The listing builds one solid part. Answer for the finished solid, in the listing's coordinates (mm). Face numbers are marked on the shaded views. A direction names the side the tool comes from. Give positions to 0.01 mm unless a question says otherwise; leave off trailing zeros. Order: outer loops, then holes, each group sorted by start corner. A loop starts at its lowest first (then second) coordinate and runs counter-clockwise, first axis right, second up. Notation, with made-up numbers: (-5, 12) - (3, 12) arc R17 ccw to (3, 24) - close; hole circle Ø4 at (14, 32). An arc over 180 degrees is marked (long way). Answer as CSV lines item,"result". Start each with the question number.
1. Consider line 1 along X through (y, z) = (-7, 52); line 2 along X through (y, z) = (4, 67.5); line 3 along Y through (x, z) = (11.1, 13.4). Determine where each line is inside the solid, lowest interval first. Write a range as [from, to].
2. Determine the mould class of the marked faces 1, 2 and 3 for opening direction X: +X half, -X half, draft (parallel to the pull), parting line (faces both ways), or undercut.
3. Section D-D on y = 7 is taken. Give the vertices of the cut face in (x, z).
4. Section A-A on z = 13.4 is taken. Give the vertices of the cut face in (x, y), and give its area (3 significant figures).
5. Section C-C on x = -6 is taken. Give the vertices of the cut face in (y, z), and give its area (3 significant figures).
6. Which of the six approach directions +Z, -Z, +X, -X, +Y, -Y give full straight-line access (tool end or side, diameter ignored) to the marked faces 4 and 5?
7. Section B-B on z = 39 is taken. Give the vertices of the cut face in (x, y).
8. Flat-ended cylindrical pins translate along their axes: pin 1 (10 mm diameter, centred on y = -3, z = 91, fed in from -X); pin 2 (7 mm diameter, centred on y = -1, z = 15.5, fed in from +X); pin 3 (1.1 mm diameter, centred on x = 13, z = 14, fed in from -Y); pin 4 (0.7 mm diameter, centred on x = 12.5, z = 13.5, fed in from +Y). Find the tip coordinate at first contact, or state that the pin passes through.
Autodesk Inventor part; units mm, degrees
ref_plane "Work Plane2" through (0, 9.7015, 84.25) normal (0.7660444, 0, 0.6427876) x (0, -1, 0)
ref_plane "YZ Plane" through (0, 0, 0) normal (1, 0, 0) x (0, 1, 0)
ref_plane "XZ Plane" through (0, 0, 0) normal (0, 1, 0) x (-1, 0, 0)
sketch "Sketch1" plane through (0, 0, 0) normal (0, 0, 1) x (1, 0, 0)
  line L0 (-12.4, 10.5) -> (12.4, 10.5)
  line L1 (12.4, 10.5) -> (12.4, -10.5)
  line L2 (12.4, -10.5) -> (-12.4, -10.5)
  line L3 (-12.4, -10.5) -> (-12.4, 10.5)
  point P0 (0, 0)
  point P1 (-12.4, 0)
  point P2 (0, 10.5)
  dimension "d0" = 24.8
  dimension "d1" = 21
extrude "Extrusion1" add sketch "Sketch1" along normal blind 1.75
ref_plane "Work Plane1" through (0, 0, 84.25) normal (0, 0, 1) x (1, 0, 0)
sketch "Sketch3" plane through (0, 0, 84.25) normal (0, 0, 1) x (1, 0, 0)
  line L0 (0, 9.7015) -> (0, -9.7015) construction
  point P0 (0, 0)
  point P1 (0, 0)
ref_plane "Work Plane2" through (0, 9.7015, 84.25) normal (0.7660444, 0, 0.6427876) x (0, -1, 0)
sketch "Sketch2" plane through (0, 0, 1.75) normal (0, 0, 1) x (1, 0, 0)
  line L0 (12.4, 10.5) -> (12.4, -10.5)
  line L1 (-12.4, 10.5) -> (12.4, 10.5)
  line L2 (12.4, -10.5) -> (-12.4, -10.5)
  line L3 (-12.4, 10.5) -> (-10.65, 10.5)
  line L4 (-10.65, 10.5) -> (-10.65, -10.5)
  line L5 (-10.65, -10.5) -> (-12.4, -10.5)
  line L6 (-12.4, -10.5) -> (-12.4, 10.5)
  line L7 (12.4, -10.5) -> (10.65, -10.5)
  line L8 (10.65, -10.5) -> (10.65, 10.5)
  line L9 (10.65, 10.5) -> (12.4, 10.5)
  line L10 (12.4, 10.5) -> (12.4, -10.5)
  point P0 (0, 0)
  dimension "d4" = 1.75
  dimension "d5" = 1.75
extrude "Extrusion2" add sketch "Sketch2" along normal up to surface contours L0 L2 L8 L1 | L4 L2 L6 L1 surface through (0, 9.7015, 84.25) normal (0.7660444, 0, 0.6427876)
sketch "Sketch4" plane through (-12.4, -10.5, 0) normal (0, -1, 0) x (1, 0, 0)
  line L0 (1.75, 96.9422) -> (0, 99.0277)
  line L1 (24.8, 69.4723) -> (23.05, 71.5578)
  line L2 (23.05, 1.75) -> (23.05, 71.5578)
  line L3 (23.05, 71.5578) -> (23.05, 74.2803)
  line L4 (23.05, 74.2803) -> (39.014, 55.2552)
  line L5 (39.014, 55.2552) -> (37.6734, 54.1303)
  line L6 (37.6734, 54.1303) -> (24.8, 69.4723)
  line L7 (0, 99.0277) -> (-12.8734, 114.3697)
  line L8 (-12.8734, 114.3697) -> (-11.5328, 115.4946)
  line L9 (-11.5328, 115.4946) -> (1.75, 99.6647)
  line L10 (1.75, 99.6647) -> (1.75, 96.9422)
  line L11 (24.8, 0) -> (24.8, 69.4723)
  line L12 (23.05, 71.5578) -> (23.05, 74.2803)
  line L13 (23.05, 74.2803) -> (1.75, 99.6647)
  line L14 (1.75, 99.6647) -> (1.75, 96.9422)
  line L15 (1.75, 96.9422) -> (23.05, 71.5578)
  point P0 (12.4, 0)
  dimension "d10" = 1.75
  dimension "d11" = 22.75
  dimension "d12" = 1.75
  dimension "d13" = 22.75
extrude "Extrusion3" add sketch "Sketch4" against normal up to surface (21 mm away)
sketch "Sketch5" plane through (-10.65, -10.5, 1.75) normal (1, 0, 0) x (0, 0, -1)
  line L0 (0, 0) -> (-95.1922, 0)
  line L1 (0, 21) -> (-23.3, 21)
  line L2 (-23.3, 21) -> (-23.3, 0)
  line L3 (-23.3, 0) -> (0, 0)
  line L4 (0, 0) -> (0, 21)
  circle A0 centre (-11.65, 10.5) radius 1.7
  point P0 (-97.7359, 0)
  point P1 (1.75, 10.5)
  dimension "d16" = 23.3
  dimension "d17" = 3.4
extrude "Extrusion4" cut sketch "Sketch5" against normal up to surface (1.75 mm away) contours A0
mirror "Mirror1" about plane through (0, 0, 0) normal (1, 0, 0) of "Extrusion4"
sketch "Sketch8" plane through (-23.9328, -10.5, 115.4946) normal (0.7660444, 0, 0.6427876) x (0.6427876, 0, -0.7660444)
  line L0 (0, 0) -> (0, 21)
  line L1 (78.6369, 0) -> (78.6369, 21)
  circle A0 centre (10.5, 10.5) radius 1.7
  circle A1 centre (68.1369, 10.5) radius 1.7
  point P0 (103.8577, 10.5)
  point P1 (0, 10.5)
  point P2 (78.6369, 10.5)
  dimension "d25" = 3.4
  dimension "d26" = 3.4
  dimension "d27" = 10.5
  dimension "d28" = 10.5
extrude "Extrusion6" cut sketch "Sketch8" against normal up to surface (1.75 mm away)
sketch "Sketch9" plane through (-12.4, -10.5, 99.0277) normal (-0.7660444, 0, -0.6427876) x (-0.6427876, 0, 0.7660444)
  circle A0 centre (9.5275, 10.5) radius 1.7
  line L0 (20.0275, 21) -> (0, 21)
  circle A1 centre (9.5275, 10.5) radius 4.3
  line L1 (11.1441, 7.7) -> (7.9109, 7.7)
  line L2 (7.9109, 7.7) -> (6.2943, 10.5)
  line L3 (6.2943, 10.5) -> (7.9109, 13.3)
  line L4 (7.9109, 13.3) -> (11.1441, 13.3)
  line L5 (11.1441, 13.3) -> (12.7606, 10.5)
  line L6 (12.7606, 10.5) -> (11.1441, 7.7)
  circle A2 centre (-48.1094, 10.5) radius 1.7
  line L7 (-38.582, 21) -> (-58.6094, 21)
  circle A3 centre (-48.1094, 10.5) radius 4.3
  line L8 (-46.4929, 7.7) -> (-49.726, 7.7)
  line L9 (-49.726, 7.7) -> (-51.3426, 10.5)
  line L10 (-51.3426, 10.5) -> (-49.726, 13.3)
  line L11 (-49.726, 13.3) -> (-46.4929, 13.3)
  line L12 (-46.4929, 13.3) -> (-44.8763, 10.5)
  line L13 (-44.8763, 10.5) -> (-46.4929, 7.7)
  point P0 (-83.8302, 10.5)
  dimension "d31" = 5.6
  dimension "d32" = 1.5
  dimension "d38" = 5.6
  dimension "d39" = 1.5
extrude "Extrusion7" cut sketch "Sketch9" against normal blind 0.75 contours L1 L2 L3 L4 L5 L6
extrude "Extrusion8" add sketch "Sketch9" along normal blind 1.55 contours A1
draft "FaceDraft1" angle 45 pull direction (-0.7660444, 0, -0.6427876) faces at (-22.0708, -0.346, 108.9453) fixed edges at (-16.9475, 0, 102.0359)
extrude "Extrusion9" cut sketch "Sketch9" against normal blind 0.75 contours L8 L9 L10 L11 L12 L13
extrude "Extrusion10" add sketch "Sketch9" along normal blind 1.55 contours A3
draft "FaceDraft2" angle 45 pull direction (-0.7660444, 0, -0.6427876) faces at (15.0044, -0.6898, 64.7609) fixed edges at (20.1008, 0, 57.8835)
sketch "Sketch10" plane through (12.4, -10.5, 0) normal (1, 0, 0) x (0, 0, -1)
  circle A0 centre (-13.4, 10.5) radius 1.7
  line L0 (0, 21) -> (-69.4723, 21)
  circle A1 centre (-13.4, 10.5) radius 4.3
  line L1 (-11.7834, 7.7) -> (-15.0166, 7.7)
  line L2 (-15.0166, 7.7) -> (-16.6332, 10.5)
  line L3 (-16.6332, 10.5) -> (-15.0166, 13.3)
  line L4 (-15.0166, 13.3) -> (-11.7834, 13.3)
  line L5 (-11.7834, 13.3) -> (-10.1668, 10.5)
  line L6 (-10.1668, 10.5) -> (-11.7834, 7.7)
  point P0 (0, 10.5)
  dimension "d45" = 5.6
  dimension "d46" = 1.5
extrude "Extrusion11" cut sketch "Sketch10" against normal blind 0.75 contours L1 L2 L3 L4 L5 L6
extrude "Extrusion12" add sketch "Sketch10" along normal blind 1.55 contours A1
draft "FaceDraft3" angle 45 pull direction (1, 0, 0) faces at (12.9167, -0.6898, 9.1557) fixed edges at (13.95, 0, 17.7)
sketch "Sketch11" plane through (-10.65, -10.5, 1.75) normal (1, 0, 0) x (0, 0, -1)
  line L0 (0, 0) -> (-95.1922, 0)
  line L1 (0, 21) -> (0, 0)
  line L2 (0, 21) -> (-95.1922, 21)
  line L3 (-25.35, 21) -> (-23.6, 21)
  line L4 (-23.6, 21) -> (-23.6, 0)
  line L5 (-23.6, 0) -> (-25.35, 0)
  line L6 (-25.35, 0) -> (-25.35, 21)
  point P0 (1.75, 10.5)
  dimension "d52" = 1.75
  dimension "d53" = 23.6
extrude "Extrusion13" add sketch "Sketch11" along normal blind 3 contours L0 L6 L2 L4
mirror "Mirror2" about plane through (0, 0, 0) normal (1, 0, 0) of "Extrusion13"
equation "\"d4\" = d5"
equation "\"d12\" = d10"
equation "\"d26\" = d25"
equation "\"d28\" = d27"
properties part number "carousel_mount_bracket"
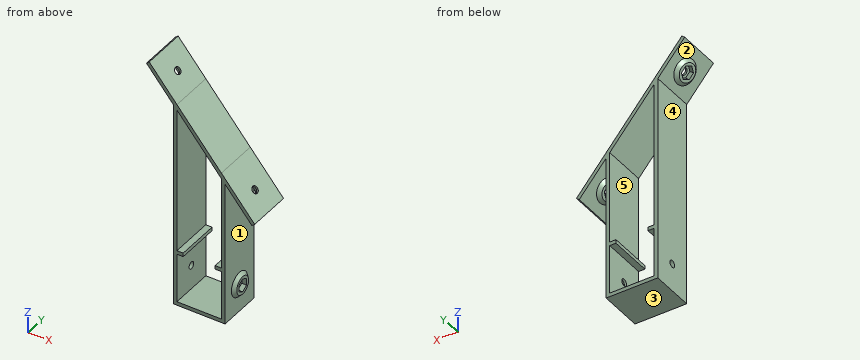
Checks:
1,line 1,"x = [-12.4, -10.65], [10.65, 12.4]"
1,line 2,"x = [-12.4, -10.65], [10.65, 12.4], [14.05, 16.34]"
1,line 3,"y = [-10.5, -1.7], [1.7, 10.5]"
2,face 1,"undercut"
2,face 2,"-X half"
2,face 3,"draft"
3,outline,"(-25.27, 114.37) - (-12.4, 99.03) - (-12.4, 0) - (12.4, 0) - (12.4, 69.47) - (25.27, 54.13) - (26.61, 55.26) - (10.65, 74.28) - (-10.65, 99.66) - (-23.93, 115.49) - close; hole (-10.65, 1.75) - (10.65, 1.75) - (10.65, 25.35) - (7.65, 25.35) - (7.65, 27.1) - (10.65, 27.1) - (10.65, 71.56) - (-10.65, 96.94) - (-10.65, 27.1) - (-7.65, 27.1) - (-7.65, 25.35) - (-10.65, 25.35) - close"
4,outline,"(-12.4, -10.5) - (-10.65, -10.5) - (-10.65, -1.7) - (-12.4, -1.7) - close; (-12.4, 1.7) - (-10.65, 1.7) - (-10.65, 10.5) - (-12.4, 10.5) - close; (10.65, -10.5) - (12.4, -10.5) - (12.4, -5.85) - (13.95, -4.3) - (13.95, -2.8) - (11.65, -2.8) - (11.65, -1.7) - (10.65, -1.7) - close; (10.65, 1.7) - (11.65, 1.7) - (11.65, 2.8) - (13.95, 2.8) - (13.95, 4.3) - (12.4, 5.85) - (12.4, 10.5) - (10.65, 10.5) - close"
4,area,"67.0 mm²"
5,outline,"(-10.5, 0) - (10.5, 0) - (10.5, 1.75) - (-10.5, 1.75) - close; (-10.5, 91.4) - (10.5, 91.4) - (10.5, 94.12) - (-10.5, 94.12) - close"
5,area,"93.9 mm²"
6,face 4,"-Z, -X, +Y, -Y"
6,face 5,"+Y, -Y"
7,outline,"(-12.4, -10.5) - (-10.65, -10.5) - (-10.65, 10.5) - (-12.4, 10.5) - close; (10.65, -10.5) - (12.4, -10.5) - (12.4, 10.5) - (10.65, 10.5) - close"
8,pin 1,"stops at x = -12.4"
8,pin 2,"stops at x = 13.95"
8,pin 3,"stops at y = -5.77"
8,pin 4,"stops at y = 10.5"
